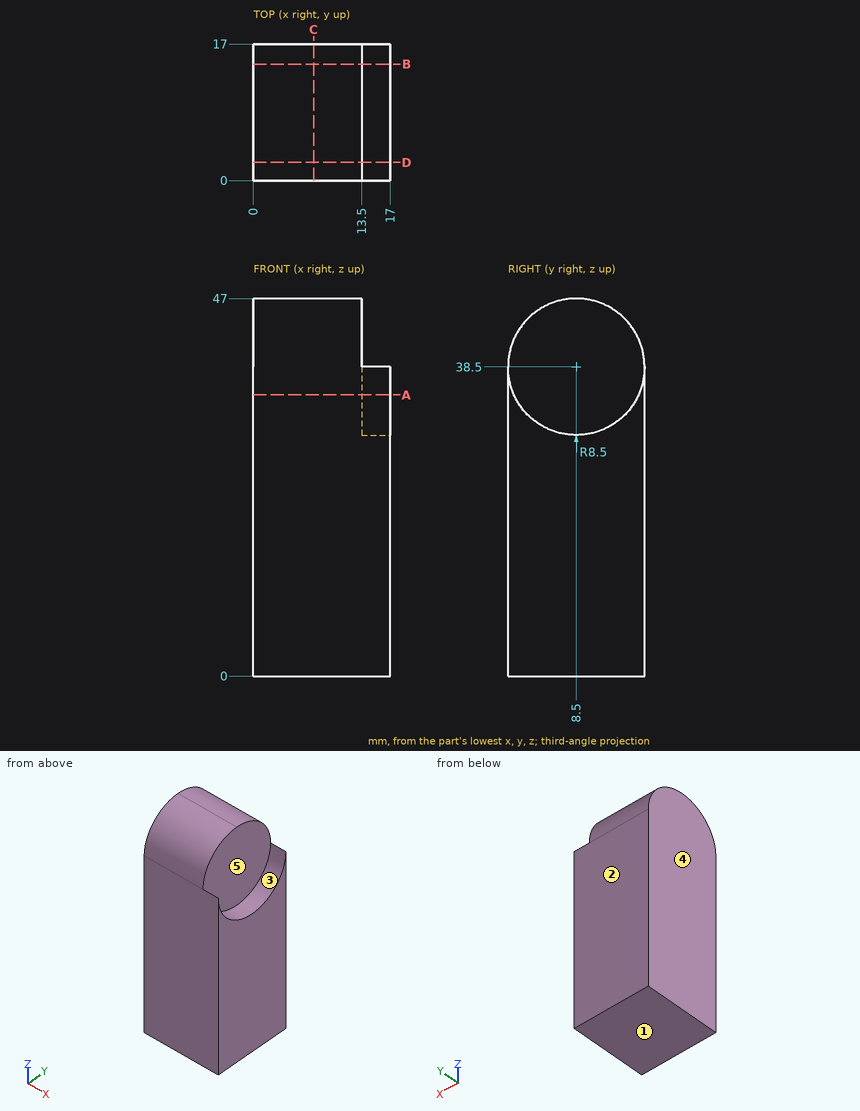
Verification items for this drawing (mm, ordinates from the low corner). A direction names the side the tool comes from. Round coordinates to 2 decimals unless told otherwise and drop trailing zeros. Order: outer loops, then holes, each group sorted by start corner. A loop starts at its lowest first (then second) coordinate and runs counter-clockwise, first axis right, second up.
1) Tool access check on the marked faces 4 and 5. Record the directions out of +Z, -Z, +X, -X, +Y, -Y that give a thin tool (end or side, any length) a straight path to the whole face; none if there is none.
Geometry says:
face 4: +Z, -Z, -X, +Y, -Y
face 5: +Z, +X
2) Draft check along Y on the marked faces 1, 2 and 3. Enter one of: +Y half, -Y half, draft (parallel to the pull), parting line (faces both ways), or undercut.
Geometry says:
face 1: draft
face 2: +Y half
face 3: undercut
3) Cross-section at C-C, the plane x = 7.5. Record the cut outline in (y, z), plus the area to 3 significant figures.
Geometry says:
outline: (0, 0) - (17, 0) - (17, 38.5) arc R8.5 ccw to (0, 38.5) - close
area: 768 mm2
4) Depth check by flat-ended pin: pin 1 (10 mm diameter, centred on x = 2.5, y = 12, fed in from +Z); pin 2 (5 mm diameter, centred on y = 11, z = 40, fed in from +X). Enter the tip coordinate at first touch or a pass-through.
Geometry says:
pin 1: stops at z = 47
pin 2: stops at x = 13.5
5) Cross-section at D-D, the plane y = 2.25. Record the cut outline in (x, z), plus the area to 3 significant figures.
Geometry says:
outline: (0, 0) - (17, 0) - (17, 32.74) - (13.5, 32.74) - (13.5, 44.26) - (0, 44.26) - close
area: 712 mm2
6) Material ranges on line 1 (X direction, y = 10.5, z = 31); line 2 (Z direction, x = 4.5, y = 3.5); line 3 (Z direction, x = 4, y = 14), recorded low to high.
Geometry says:
line 1: x = 0 to 13.5
line 2: z = 0 to 45.37
line 3: z = 0 to 44.98
7) Cross-section at A-A, the plane z = 35. Record the cut outline in (x, y).
Geometry says:
outline: (0, 0) - (17, 0) - (17, 0.75) - (13.5, 0.75) - (13.5, 16.25) - (17, 16.25) - (17, 17) - (0, 17) - close
8) Cross-section at B-B, the plane y = 14.5. Record the cut outline in (x, z).
Geometry says:
outline: (0, 0) - (17, 0) - (17, 32.48) - (13.5, 32.48) - (13.5, 44.52) - (0, 44.52) - close
